Part print with two shaded views. Sizes in mm from the minimum x, y, z corner. Round coordinates to 2 decimals unless told otherwise and drop trailing zeros. Loops run counter-clockwise (first coordinate to the right, second up) from the corner with the lowest first, then second, coordinate; pieces in that order, holes last. Notation, with made-up numbers: (-32, 87) - (-18, 87) arc R8 cw to (-18, 95) - close; hole circle Ø2 at (21, -33). An arc over 180 degrees is marked (long way). Use a Markdown table: item, result.
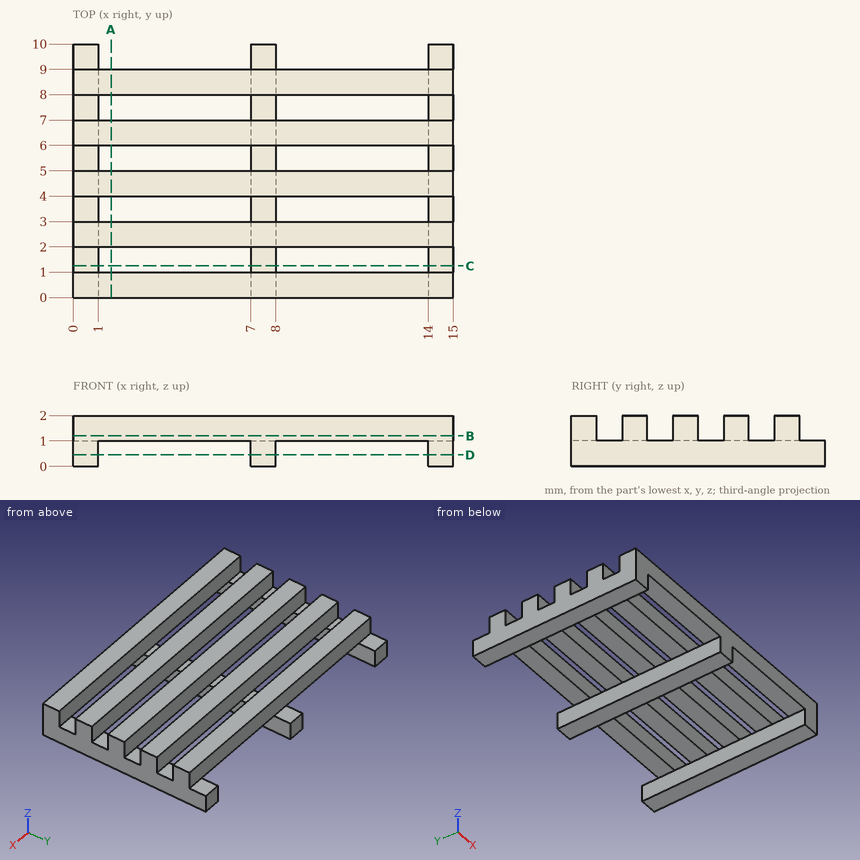
Q1. Cut at B-B, the plane z = 1.2. List the corners of the cut face in (x, y), plus the area to 3 significant figures.
Results found:
| item | result |
|---|---|
| outline | (0, 0) - (15, 0) - (15, 1) - (0, 1) - close; (0, 2) - (15, 2) - (15, 3) - (0, 3) - close; (0, 4) - (15, 4) - (15, 5) - (0, 5) - close; (0, 6) - (15, 6) - (15, 7) - (0, 7) - close; (0, 8) - (15, 8) - (15, 9) - (0, 9) - close |
| area | 75.0 mm2 |
Q2. Cut at A-A, the plane x = 1.5. List the corners of the cut face in (y, z), plus the area to 3 significant figures.
Results found:
| item | result |
|---|---|
| outline | (0, 1) - (1, 1) - (1, 2) - (0, 2) - close; (2, 1) - (3, 1) - (3, 2) - (2, 2) - close; (4, 1) - (5, 1) - (5, 2) - (4, 2) - close; (6, 1) - (7, 1) - (7, 2) - (6, 2) - close; (8, 1) - (9, 1) - (9, 2) - (8, 2) - close |
| area | 5.00 mm2 |
Q3. Drop flat-ended pins along their axis: pin 1 (0.8 mm diameter, centred on x = 7.5, y = 5.5, fed in from +Z); pin 2 (0.5 mm diameter, centred on x = 5, y = 4.5, fed in from -Z); pin 3 (0.5 mm diameter, centred on x = 6, z = 1.5, fed in from +Y). Give the stop position or say it passes through.
Results found:
| item | result |
|---|---|
| pin 1 | stops at z = 1 |
| pin 2 | stops at z = 1 |
| pin 3 | stops at y = 9 |
Q4. Probe line 1 (Y direction, x = 13, z = 1.5); line 2 (X direction, y = 5, z = 0.8); line 3 (Z direction, x = 5.25, y = 2.75). List the from-to ranges inside material, lowest first.
Results found:
| item | result |
|---|---|
| line 1 | y = 0 to 1, 2 to 3, 4 to 5, 6 to 7, 8 to 9 |
| line 2 | x = 0 to 1, 7 to 8, 14 to 15 |
| line 3 | z = 1 to 2 |
Q5. Cut at C-C, the plane y = 1.25. List the corners of the cut face in (x, z).
Results found:
| item | result |
|---|---|
| outline | (0, 0) - (1, 0) - (1, 1) - (0, 1) - close; (7, 0) - (8, 0) - (8, 1) - (7, 1) - close; (14, 0) - (15, 0) - (15, 1) - (14, 1) - close |
Q6. Cut at D-D, the plane z = 0.45. List the corners of the cut face in (x, y), plus the area to 3 significant figures.
Results found:
| item | result |
|---|---|
| outline | (0, 0) - (1, 0) - (1, 10) - (0, 10) - close; (7, 0) - (8, 0) - (8, 10) - (7, 10) - close; (14, 0) - (15, 0) - (15, 10) - (14, 10) - close |
| area | 30.0 mm2 |
